For this review, use the dimensioned drawing (mm, ordinates from the lowest corner) and the shaded views. Coordinates: 2 decimals unless noted, no trailing zeros. Loops run counter-clockwise (first coordinate to the right, second up) from the corner with the lowest first, then second, coordinate; pieces in that order, holes last. Notation, with made-up numbers: (89.5, -17) - (99.5, -17) arc R12 ccw to (99.5, 3) - close; hole circle Ø5 at (-19, 10). An arc over 180 degrees is marked (long way). Return JSON: item names as keys, results as strings. Group by question number.
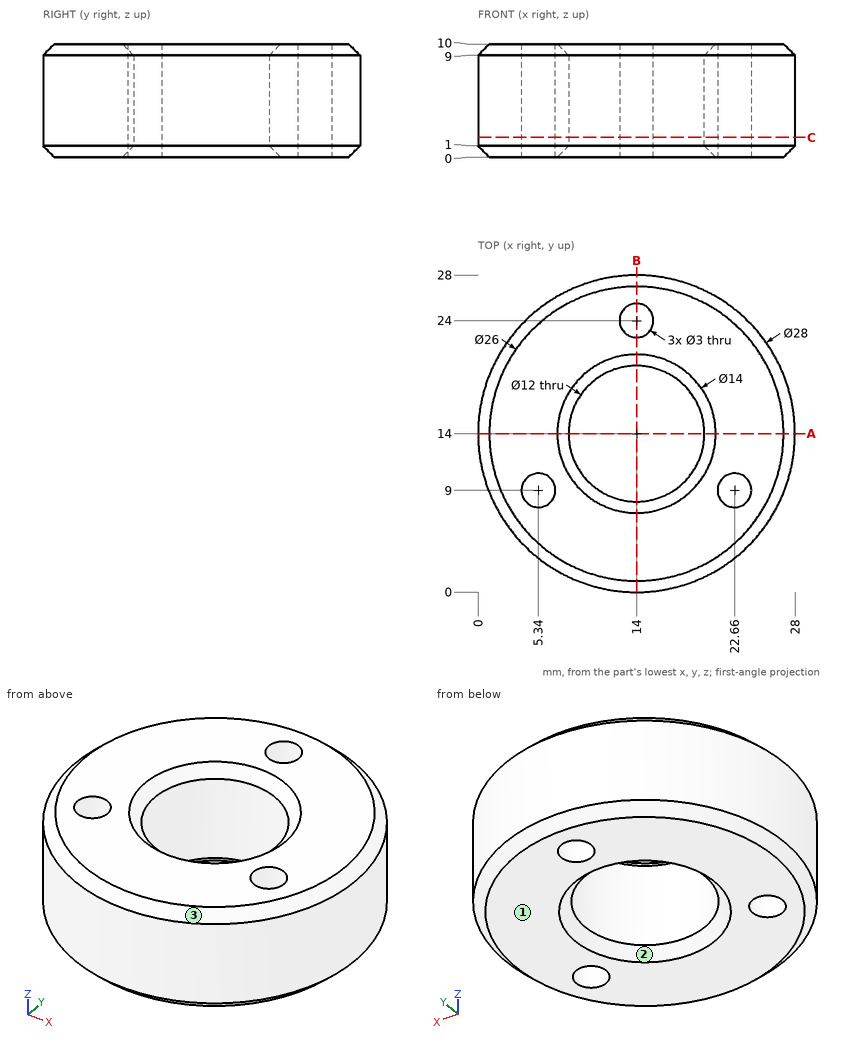
Item 1: To check wall thickness, follow line 1 (Y direction, x = 14, z = 5.25); line 2 (Y direction, x = 12.75, z = 7.25) (1 decimal); line 3 (Y direction, x = 23.75, z = 5). State the ranges of each line that lie inside material, in increasing order. Write a range as from..to.
Item 2: Draft analysis for pull direction X (two halves, no side actions). For the marked faces 1, 2 and 3, state which applies: pulls with the +X half, pulls with the -X half, needs draft (parallel to the pull), parting line crosses it, or undercut.
Item 3: Add section A-A (y = 14). State the section outline as (x, z) points.
Item 4: For P1, Ø2, axis at x = 17, z = 4.5, coming from the +Y side; P2, Ø12, axis at x = 19.5, y = 6, coming from the -Z side; P3, Ø4, axis at x = 24.5, z = 8, coming from the -Y side (1 decimal), all flat-tipped, find the tip position at first contact; note any pin that passes through.
Item 5: Add section C-C (z = 1.75). State the section outline as (x, y) points.
Item 6: Add section B-B (x = 14). State the section outline as (y, z) points.
Answers below:
{
 "1": {"line 1": "y = 0..8, 20..22.5, 25.5..28", "line 2": "y = 0.1..8.1, 19.9..23.2, 24.8..27.9", "line 3": "y = 3.95..7.97, 10.03..24.05"},
 "2": {"face 1": "needs draft", "face 2": "undercut", "face 3": "parting line crosses it"},
 "3": {"outline": "(0, 1) - (1, 0) - (7, 0) - (8, 1) - (8, 9) - (7, 10) - (1, 10) - (0, 9) - close; (20, 1) - (21, 0) - (27, 0) - (28, 1) - (28, 9) - (27, 10) - (21, 10) - (20, 9) - close"},
 "4": {"P1": "stops at y = 27.86", "P2": "stops at z = 0", "P3": "stops at y = 2.9"},
 "5": {"outline": "circle Ø28 at (14, 14); hole circle Ø3 at (5.34, 9); hole circle Ø12 at (14, 14); hole circle Ø3 at (14, 24); hole circle Ø3 at (22.66, 9)"},
 "6": {"outline": "(0, 1) - (1, 0) - (7, 0) - (8, 1) - (8, 9) - (7, 10) - (1, 10) - (0, 9) - close; (20, 1) - (21, 0) - (22.5, 0) - (22.5, 10) - (21, 10) - (20, 9) - close; (25.5, 0) - (27, 0) - (28, 1) - (28, 9) - (27, 10) - (25.5, 10) - close"}
}
